Verification items for the finished model (mm, model axes). A direction names the side the tool comes from. Round coordinates to 2 decimals unless told otherwise and drop trailing zeros. Loops run counter-clockwise (first coordinate to the right, second up) from the corner with the lowest first, then second, coordinate; pieces in that order, holes last. Notation, with made-up numbers: M 46,-39.75 L 88,-39.75 A18 ccw 88,-20.75 Z; hole C 72.5,56 d9. An arc over 180 degrees is marked long. One line per item, written item: value.
from build123d import *

# Parameters (mm, degrees)
SKETCH1_R           = 6
BOSS_EXTRUDE1_DEPTH = 40
SKETCH2_R           = 9
BOSS_EXTRUDE2_DEPTH = 25
SKETCH4_R           = 3
CUT_EXTRUDE1_DEPTH  = 45
SKETCH6_R           = 3
CUT_EXTRUDE2_DEPTH  = 10


with BuildPart() as part:
    # Sketch1 → Boss-Extrude1 (new body, symmetric)
    with BuildSketch(Plane.XY):
        Circle(SKETCH1_R)
    extrude(amount=BOSS_EXTRUDE1_DEPTH, both=True)

    # Sketch2 → Boss-Extrude2 (add, symmetric)
    with BuildSketch(Plane.XY):
        Circle(SKETCH2_R)
    extrude(amount=BOSS_EXTRUDE2_DEPTH, both=True)

    # Sketch4 → Cut-Extrude1 (cut)
    with BuildSketch(Plane.XY.offset(40)):
        Circle(SKETCH4_R)
    extrude(amount=-CUT_EXTRUDE1_DEPTH, mode=Mode.SUBTRACT)

    # Sketch6 → Cut-Extrude2 (cut, through all)
    with BuildSketch(Plane(origin=(0, 0, 0), x_dir=(0, 0, -1), z_dir=(1, 0, 0))):
        Circle(SKETCH6_R)
    extrude(amount=-CUT_EXTRUDE2_DEPTH, mode=Mode.SUBTRACT)


solid = part.part
(1) Tool access check on faces 4 (the face through (-3, -1, 40)), 5 (the face through (0, 0, -40)), 6 (the face through (-5, 0, 3)), 7 (the face through (-6, 0, -32)), 8 (the face through (0, 0, -5)). Record the directions out of +Z, -Z, +X, -X, +Y, -Y that give a thin tool (end or side, any length) a straight path to the whole face; none if there is none.
Completed:
face 4: +Z, +X, -X, +Y, -Y
face 5: -Z, +X, -X, +Y, -Y
face 6: -X
face 7: -Z
face 8: +Z
(2) Mould release check, pull along Y, two halves, no side actions. Record for faces 1 (the face through (2, -6, 25)), 2 (the face through (-6, 0, 33)), 3 (the face through (2.77, -1.15, 17.82)): +Y half, -Y half, draft (parallel to the pull), parting line (faces both ways), or undercut.
Completed:
face 1: draft
face 2: parting line
face 3: undercut
(3) Thickness scan on L1, parallel to Y at x = 0, z = 26; L2, parallel to Y at x = 0, z = 19; L3, parallel to Z at x = -2.5, y = 0. Record the ranges inside material, lowest first. Write a range as from..to.
Completed:
L1: y = -6..-3, 3..6
L2: y = -9..-3, 3..9
L3: z = -40..-5
(4) Sectioned sample at A-A on y = 0. Enter the section's corners in (x, z), and give its area (3 significant figures).
Completed:
outline: M -9,-25 L -6,-25 L -6,-40 L 6,-40 L 6,-25 L 9,-25 L 9,25 L 6,25 L 6,40 L 3,40 L 3,-5 L -3,-5 L -3,-3 L -9,-3 Z; M -9,3 L -3,3 L -3,40 L -6,40 L -6,25 L -9,25 Z
area: 954 mm^2
(5) Sectioned sample at D-D on y = 5. Enter the section's corners in (x, z).
Completed:
outline: M -7.48,-25 L -3.32,-25 L -3.32,-40 L 3.32,-40 L 3.32,-25 L 7.48,-25 L 7.48,25 L 3.32,25 L 3.32,40 L -3.32,40 L -3.32,25 L -7.48,25 Z
(6) Depth check by flat-ended pin: pin 1 Ø2 at (y, z) = (7, -4.5) entering from -X; pin 2 Ø5 at (x, z) = (3, -24) entering from -Y; pin 3 Ø5 at (x, y) = (-7, 5.5) entering from +Z. Enter the tip coordinate at first touch or a pass-through.
Completed:
pin 1: stops at x = -6.71
pin 2: stops at y = -8.99
pin 3: stops at z = 25
(7) Sectioned sample at B-B on x = -5. Enter the section's corners in (y, z).
Completed:
outline: M -7.48,-25 L -3.32,-25 L -3.32,-40 L 3.32,-40 L 3.32,-25 L 7.48,-25 L 7.48,25 L 3.32,25 L 3.32,40 L -3.32,40 L -3.32,25 L -7.48,25 Z; hole C 0,0 d6
(8) Sectioned sample at C-C on z = 22. Enter the section's corners in (x, y).
Completed:
outline: C 0,0 d18; hole C 0,0 d6
